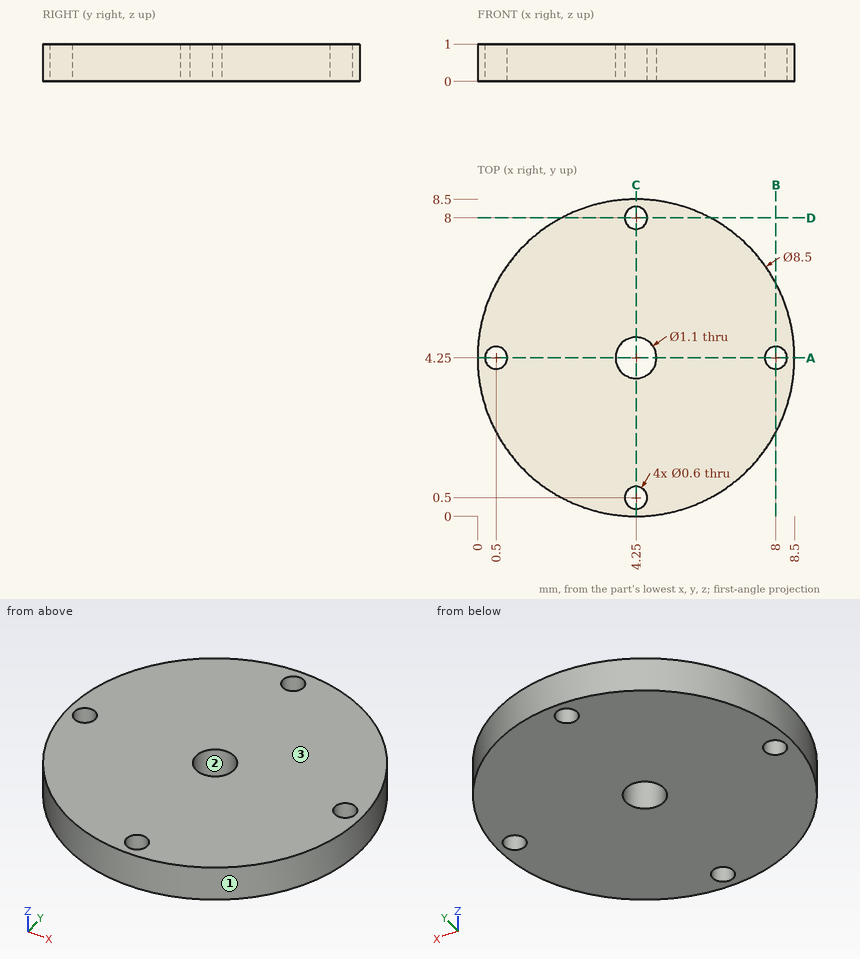
Part print with two shaded views. Sizes in mm from the minimum x, y, z corner. Coordinates: 2 decimals unless noted, no trailing zeros. Write each loop counter-clockwise with the first axis right and the second up, starting at its lowest first coordinate (ties: lowest second). Pieces come first, ordered by that corner, then holes. Notation, with made-up numbers: (-0.75, 59.5) -> (27.25, 59.5) arc R24 cw to (27.25, 87.5) -> close; hole circle Ø4 at (85, 73). An arc over 180 degrees is marked (long way). Return JSON: item names as keys, results as strings. Group by question number.
Q1. Cut at A-A, the plane y = 4.25. Give the cut face in (x, z).
Q2. Cut at B-B, the plane x = 8. Give the cut face in (y, z), then the cut area to 3 significant figures.
Q3. Flat gauge pin, fed straight in: pin 1 (0.9 mm diameter, centred on x = 4.25, y = 4.25, fed in from -Z). Where does the tip first touch, or does it go through?
Q4. Drill centre lines: line 1 (Y direction, x = 4.25, z = 0.35); line 2 (Y direction, x = 0.5, z = 0.1); line 3 (X direction, y = 2, z = 0.4). Where is each one in solid material? Low to high.
Q5. Pull direction X, two halves, no side cores. Call the marked faces 1, 2 and 3: released by +X, released by -X, zero draft, split by the parting line, or undercut.
Returned:
{
 "1": {"outline": "(0, 0) -> (0.2, 0) -> (0.2, 1) -> (0, 1) -> close; (0.8, 0) -> (3.7, 0) -> (3.7, 1) -> (0.8, 1) -> close; (4.8, 0) -> (7.7, 0) -> (7.7, 1) -> (4.8, 1) -> close; (8.3, 0) -> (8.5, 0) -> (8.5, 1) -> (8.3, 1) -> close"},
 "2": {"outline": "(2.25, 0) -> (3.95, 0) -> (3.95, 1) -> (2.25, 1) -> close; (4.55, 0) -> (6.25, 0) -> (6.25, 1) -> (4.55, 1) -> close", "area": "3.40 mm2"},
 "3": {"pin 1": "passes through"},
 "4": {"line 1": "y = 0 to 0.2, 0.8 to 3.7, 4.8 to 7.7, 8.3 to 8.5", "line 2": "y = 2.25 to 3.95, 4.55 to 6.25", "line 3": "x = 0.64 to 7.86"},
 "5": {"face 1": "split by the parting line", "face 2": "undercut", "face 3": "zero draft"}
}
